from build123d import *

# Parameters (mm, degrees)
F1_DEPTH = 7
F2_DEPTH = 3
F3_DEPTH = 3


# Not quite as in the source:
# - a feature names something its author has since deleted; it is built from what else it names


with BuildPart() as f1:
    # F0 (on Top) → F1 (new body)
    with BuildSketch(Plane.XY):
        with BuildLine():
            Line((-1.1851356201, 23.1923339907), (-5.6851356201, 23.1923339907))
            ThreePointArc((-5.6851356201, 23.1923339907), (-3.6139055058, 21.83796352), (-1.1851356201, 21.3632105309))
            Line((-1.1851356201, 21.3632105309), (-1.1851356201, 23.1923339907))
        make_face()
        with BuildLine():
            ThreePointArc((-1.1851356201, 21.3632105309), (1.2436342657, 21.83796352), (3.3148643799, 23.1923339907))
            Line((3.3148643799, 23.1923339907), (-1.1851356201, 23.1923339907))
            Line((-1.1851356201, 23.1923339907), (-1.1851356201, 21.3632105309))
        make_face()
        with BuildLine():
            ThreePointArc((-7.6351356201, 27.8132105309), (-7.1276729569, 25.3054725063), (-5.6851356201, 23.1923339907))
            Line((-5.6851356201, 23.1923339907), (-1.1851356201, 23.1923339907))
            Line((-1.1851356201, 23.1923339907), (-1.1851356201, 25.8132105309))
            ThreePointArc((-1.1851356201, 25.8132105309), (-2.5993491824, 26.3989969686), (-3.1851356201, 27.8132105309))
            Line((-3.1851356201, 27.8132105309), (-7.6351356201, 27.8132105309))
        make_face()
        with BuildLine():
            Line((-1.1851356201, 23.1923339907), (3.3148643799, 23.1923339907))
            ThreePointArc((3.3148643799, 23.1923339907), (4.7574017168, 25.3054725063), (5.2648643799, 27.8132105309))
            Line((5.2648643799, 27.8132105309), (0.8148643799, 27.8132105309))
            ThreePointArc((0.8148643799, 27.8132105309), (0.2290779423, 26.3989969686), (-1.1851356201, 25.8132105309))
            Line((-1.1851356201, 25.8132105309), (-1.1851356201, 23.1923339907))
        make_face()
        with BuildLine():
            Line((-5.0348369716, 18.4756626995), (-3.9452707751, 10.572946599))
            ThreePointArc((-3.9452707751, 10.572946599), (-3.2076275018, 12.6510857986), (-1.1851356201, 13.5298956301))
            Line((-1.1851356201, 13.5298956301), (-1.1851356201, 17.7132105309))
            ThreePointArc((-1.18513562, 17.7132105309), (-3.1473750171, 17.9056570212), (-5.0348369716, 18.4756626995))
        make_face()
        with BuildLine():
            ThreePointArc((-3.9452707751, 10.572946599), (-1.0899472994, 7.9981634027), (1.5815494791, 10.7632105309))
            ThreePointArc((1.5815494791, 10.7632105309), (1.5769058667, 10.923439316), (1.562990617, 11.0831302441))
            ThreePointArc((1.562990617, 11.0831302441), (0.6546237847, 12.8295676566), (-1.1851356201, 13.5298956301))
            ThreePointArc((-1.1851356201, 13.5298956301), (-3.2076275018, 12.6510857986), (-3.9452707751, 10.572946599))
        make_face()
        with BuildLine():
            Line((-5.3833250343, 21.0032761963), (-5.0348369716, 18.4756626995))
            ThreePointArc((-5.0348369716, 18.4756626995), (-3.1473750171, 17.9056570212), (-1.18513562, 17.7132105309))
            Line((-1.1851356201, 17.7132105309), (-1.1851356201, 19.8132105309))
            ThreePointArc((-1.1851356201, 19.8132105309), (-3.3669382375, 20.1164750321), (-5.3833250343, 21.0032761963))
        make_face()
        with BuildLine():
            Line((-5.6851356201, 23.1923339907), (-5.3833250343, 21.0032761963))
            ThreePointArc((-5.3833250343, 21.0032761963), (-3.3669382375, 20.1164750321), (-1.1851356201, 19.8132105309))
            Line((-1.1851356201, 19.8132105309), (-1.1851356201, 21.3632105309))
            ThreePointArc((-1.1851356201, 21.3632105309), (-3.6139055058, 21.83796352), (-5.6851356201, 23.1923339907))
        make_face()
        with BuildLine():
            ThreePointArc((-1.1851356201, 13.5298956301), (0.6546237847, 12.8295676566), (1.562990617, 11.0831302441))
            Line((1.562990617, 11.0831302441), (2.630466448, 18.461676921))
            ThreePointArc((2.630466448, 18.461676921), (0.7590236506, 17.9020933018), (-1.18513562, 17.7132105309))
            Line((-1.1851356201, 17.7132105309), (-1.1851356201, 13.5298956301))
        make_face()
        with BuildLine():
            ThreePointArc((-1.18513562, 17.7132105309), (0.7590236506, 17.9020933018), (2.630466448, 18.461676921))
            Line((2.630466448, 18.461676921), (2.9967135721, 20.993229788))
            ThreePointArc((2.9967135721, 20.993229788), (0.9874382057, 20.1138649112), (-1.1851356201, 19.8132105309))
            Line((-1.1851356201, 19.8132105309), (-1.1851356201, 17.7132105309))
        make_face()
        with BuildLine():
            ThreePointArc((-1.1851356201, 19.8132105309), (0.9874382057, 20.1138649112), (2.9967135721, 20.993229788))
            Line((2.9967135721, 20.993229788), (3.3148643799, 23.1923339907))
            ThreePointArc((3.3148643799, 23.1923339907), (1.2436342657, 21.83796352), (-1.1851356201, 21.3632105309))
            Line((-1.1851356201, 21.3632105309), (-1.1851356201, 19.8132105309))
        make_face()
        with BuildLine():
            Line((0.8148643799, 27.8132105309), (5.2648643799, 27.8132105309))
            ThreePointArc((5.2648643799, 27.8132105309), (-1.1851356201, 34.2632105309), (-7.6351356201, 27.8132105309))
            Line((-7.6351356201, 27.8132105309), (-3.1851356201, 27.8132105309))
            ThreePointArc((-3.1851356201, 27.8132105309), (-1.1851356201, 29.8132105309), (0.8148643799, 27.8132105309))
        make_face()
    extrude(amount=F1_DEPTH)

    # F0 (on Top) → F2 (join)
    with BuildSketch(Plane.XY):
        with BuildLine():
            Line((2.9967135721, 20.993229788), (2.630466448, 18.461676921))
            ThreePointArc((2.630466448, 18.461676921), (7.1978107858, 22.179720533), (8.9148643799, 27.8132105309))
            ThreePointArc((8.9148643799, 27.8132105309), (-6.8033211078, 36.2064215866), (-5.0348369716, 18.4756626995))
            Line((-5.0348369716, 18.4756626995), (-5.3833250343, 21.0032761963))
            ThreePointArc((-5.3833250343, 21.0032761963), (-7.8303759033, 23.3589113068), (-9.0795106201, 26.5175086519))
            ThreePointArc((-9.0795106201, 26.5175086519), (-10.4851356201, 27.8132105309), (-9.0795106201, 29.10891241))
            ThreePointArc((-9.0795106201, 29.10891241), (-6.8419898695, 33.4700647804), (-2.4808374991, 35.7075855309))
            ThreePointArc((-2.4808374991, 35.7075855309), (-1.237991827, 37.1121355562), (0.1148643799, 35.8132105309))
            ThreePointArc((0.1148643799, 35.8132105309), (0.1137894053, 35.7603543239), (0.110566259, 35.7075855309))
            ThreePointArc((0.110566259, 35.7075855309), (4.4752873931, 33.4664937639), (6.7108684576, 29.0989475203))
            ThreePointArc((6.7108684576, 29.0989475203), (7.6965647575, 28.7584108036), (8.1148580079, 27.803113359))
            ThreePointArc((8.1148580079, 27.803113359), (7.6953583299, 26.8467038322), (6.7075977264, 26.5075458262))
            ThreePointArc((6.7075977264, 26.5075458262), (5.4519425182, 23.3467584953), (2.9967135721, 20.993229788))
        make_face()
        with BuildLine():
            ThreePointArc((-9.0795106201, 26.5175086519), (-7.8303759033, 23.3589113068), (-5.3833250343, 21.0032761963))
            Line((-5.3833250343, 21.0032761963), (-5.6851356201, 23.1923339907))
            ThreePointArc((-5.6851356201, 23.1923339907), (-7.1276729569, 25.3054725063), (-7.6351356201, 27.8132105309))
            Line((-7.6351356201, 27.8132105309), (-7.8851356201, 27.8132105309))
            ThreePointArc((-7.8851356201, 27.8132105309), (-8.229281944, 26.9321068197), (-9.0795106201, 26.5175086519))
        make_face()
    extrude(amount=F2_DEPTH)

    # F0 (on Top) → F3 (join)
    with BuildSketch(Plane.XY):
        with BuildLine():
            Line((3.3148643799, 23.1923339907), (2.9967135721, 20.993229788))
            ThreePointArc((2.9967135721, 20.993229788), (5.4519425182, 23.3467584953), (6.7075977264, 26.5075458262))
            ThreePointArc((6.7075977264, 26.5075458262), (5.8555856645, 26.9257328422), (5.5148855907, 27.81158181))
            Line((5.5148855907, 27.81158181), (5.2648643799, 27.8132105309))
            ThreePointArc((5.2648643799, 27.8132105309), (4.7574017168, 25.3054725063), (3.3148643799, 23.1923339907))
        make_face()
        with BuildLine():
            ThreePointArc((-7.6351356201, 27.8132105309), (-1.1851356201, 34.2632105309), (5.2648643799, 27.8132105309))
            Line((5.2648643799, 27.8132105309), (5.5148855907, 27.81158181))
            ThreePointArc((5.5148855907, 27.81158181), (5.8624374498, 28.6879269442), (6.7108684576, 29.0989475203))
            ThreePointArc((6.7108684576, 29.0989475203), (4.4752873931, 33.4664937639), (0.110566259, 35.7075855309))
            ThreePointArc((0.110566259, 35.7075855309), (-1.1851356201, 34.5132105309), (-2.4808374991, 35.7075855309))
            ThreePointArc((-2.4808374991, 35.7075855309), (-6.8419898695, 33.4700647804), (-9.0795106201, 29.10891241))
            ThreePointArc((-9.0795106201, 29.10891241), (-8.229281944, 28.6943142422), (-7.8851356201, 27.8132105309))
            Line((-7.8851356201, 27.8132105309), (-7.6351356201, 27.8132105309))
        make_face()
    extrude(amount=F3_DEPTH)


solid = f1.part
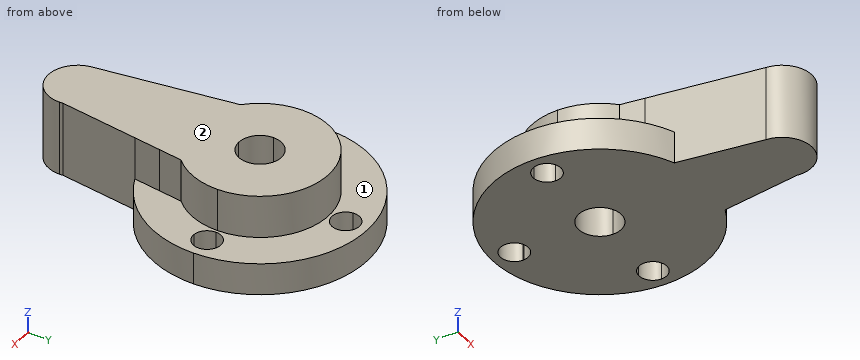
Could you check a few things on this model? Use its own coordinates, in mm. Face numbers are marked on the shaded views. A direction names the side the tool comes from. Coordinates: 2 decimals unless noted, no trailing zeros. Order: outer loops, then holes, each group sorted by start corner. A loop starts at its lowest first (then second) coordinate and runs counter-clockwise, first axis right, second up. Notation, with made-up numbers: (-12.75, 80) -> (40.25, 80) arc R19 ccw to (40.25, 108) -> close; hole circle Ø6 at (-38, -11.75). An arc over 180 degrees is marked (long way). One line per item, written item: value. Start each with the question number.
1) Imagine slicing it at C-C on z = 1.25. List the corners of the cut face in (x, y) for me.
2) Imagine slicing it at B-B on y = 35.25. List the corners of the cut face in (x, z) for me, plus the area to 3 significant figures.
3) If I drill on L1, parallel to Z at x = 3.5, y = 21; L2, parallel to Y at x = 0.25, z = 1.25; L3, parallel to X at y = 27, z = 5.75, over which ranges is the centre line in solid material (lowest first)? Write a range as [from, to].
4) Which directions (+Z, -Z, +X, -X, +Y, -Y) give clear straight access to the entire face, cutting with the end or side of a thin tool? Please do the marked faces 1 and 2.
5) Imagine slicing it at A-A on z = 6.25. List the corners of the cut face in (x, y) for me.
6) I'm going to push flat-ended pins straight in: pin 1 (1.5 mm diameter, centred on x = -5, z = 4.5, fed in from +Y); pin 2 (1 mm diameter, centred on x = -2.5, z = 4.5, fed in from +Y); pin 3 (4 mm diameter, centred on x = -9.19, y = 27.81, fed in from +Z); pin 4 (3 mm diameter, centred on y = 20, z = 6, fed in from -X). Where does each tip first touch, or does it pass through?
7) Imagine slicing it at D-D on y = 24.75. List the corners of the cut face in (x, z) for me, plus the area to 3 significant figures.
Answer list:
1. outline: (-5.03, 18.48) -> (-3.95, 10.57) arc R2.77 ccw (long way) to (1.56, 11.08) -> (2.63, 18.46) arc R10.1 ccw (long way) to start; hole circle Ø2.6 at (-9.19, 27.81); hole circle Ø4 at (-1.19, 27.81); hole circle Ø2.6 at (-1.19, 35.81); hole circle Ø2.6 at (6.81, 27.8)
2. outline: (-8.02, 0) -> (-2.36, 0) -> (-2.36, 3) -> (-8.02, 3) -> close; (-0.01, 0) -> (5.65, 0) -> (5.65, 3) -> (-0.01, 3) -> close
2. area: 34.0 mm2
3. L1: z = [0, 3]
3. L2: y = [8.4, 26.42], [29.21, 37.81]
3. L3: x = [-7.58, -3.01], [0.64, 5.21]
4. face 1: +Z
4. face 2: +Z, +X, -X, +Y, -Y
5. outline: (-5.69, 23.19) -> (-3.95, 10.57) arc R2.77 ccw (long way) to (1.56, 11.08) -> (3.31, 23.19) arc R6.45 ccw (long way) to start; hole circle Ø4 at (-1.19, 27.81)
6. pin 1: stops at y = 33.49
6. pin 2: stops at y = 34.21
6. pin 3: stops at z = 7
6. pin 4: stops at x = -5.45
7. outline: (-10.81, 0) -> (8.44, 0) -> (8.44, 3) -> (4.49, 3) -> (4.49, 7) -> (-6.86, 7) -> (-6.86, 3) -> (-10.81, 3) -> close
7. area: 103 mm2
